Verification items for the finished model (mm, model axes). Give positions to 0.01 mm unless a question says otherwise; leave off trailing zeros. Loops run counter-clockwise (first coordinate to the right, second up) from the corner with the lowest first, then second, coordinate; pieces in that order, holes last. Notation, with made-up numbers: (50, -27) - (64, -27) arc R19 ccw to (64, 7) - close; hole circle Ø7 at (5.25, -32.5). An arc over 180 degrees is marked (long way). Use one line per item in the form item = value.
```python
from build123d import *

# Parameters (mm, degrees)
SKETCH_1_R      = 80.33713036
SKETCH_1_R_2    = 4.1
EXTRUDE_1_DEPTH = 8


with BuildPart() as part:
    # 草图1 → 凸台-拉伸1 (new body)
    with BuildSketch(Plane.XY):
        Circle(SKETCH_1_R)
        with Locations((0, 73.60266962)):
            Circle(SKETCH_1_R_2, mode=Mode.SUBTRACT)
        with Locations((-52.044946802, 52.044946802)):
            Circle(SKETCH_1_R_2, mode=Mode.SUBTRACT)
        with Locations((-73.60266962, 0)):
            Circle(SKETCH_1_R_2, mode=Mode.SUBTRACT)
        with Locations((-52.044946802, -52.044946802)):
            Circle(SKETCH_1_R_2, mode=Mode.SUBTRACT)
        with Locations((0, -73.60266962)):
            Circle(SKETCH_1_R_2, mode=Mode.SUBTRACT)
        with Locations((52.044946802, -52.044946802)):
            Circle(SKETCH_1_R_2, mode=Mode.SUBTRACT)
        with Locations((73.60266962, 0)):
            Circle(SKETCH_1_R_2, mode=Mode.SUBTRACT)
        with Locations((52.044946802, 52.044946802)):
            Circle(SKETCH_1_R_2, mode=Mode.SUBTRACT)
        with Locations((0, 26.022473401)):
            Circle(SKETCH_1_R_2, mode=Mode.SUBTRACT)
        with Locations((22.536123034, -13.0112367)):
            Circle(SKETCH_1_R_2, mode=Mode.SUBTRACT)
        with Locations((-22.536123034, -13.0112367)):
            Circle(SKETCH_1_R_2, mode=Mode.SUBTRACT)
        Circle(SKETCH_1_R_2, mode=Mode.SUBTRACT)
        with BuildLine():
            Line((43.72373161, 48.096104771), (30, 33))
            Line((30, 33), (-30, 33))
            Line((-30, 33), (-43.72373161, 48.096104771))
            ThreePointArc((-43.72373161, 48.096104771), (0, 65), (43.72373161, 48.096104771))
        make_face(mode=Mode.SUBTRACT)
        with BuildLine():
            Line((-64.926428952, -3.091734712), (-44.547727215, -2.121320344))
            Line((-44.547727215, -2.121320344), (-2.121320344, -44.547727215))
            Line((-2.121320344, -44.547727215), (-3.091734712, -64.926428952))
            ThreePointArc((-3.091734712, -64.926428952), (-45.961940777, -45.961940777), (-64.926428952, -3.091734712))
        make_face(mode=Mode.SUBTRACT)
        with BuildLine():
            Line((3.091734712, -64.926428952), (2.121320344, -44.547727215))
            Line((2.121320344, -44.547727215), (44.547727215, -2.121320344))
            Line((44.547727215, -2.121320344), (64.926428952, -3.091734712))
            ThreePointArc((64.926428952, -3.091734712), (45.961940777, -45.961940777), (3.091734712, -64.926428952))
        make_face(mode=Mode.SUBTRACT)
    extrude(amount=EXTRUDE_1_DEPTH)


solid = part.part
```
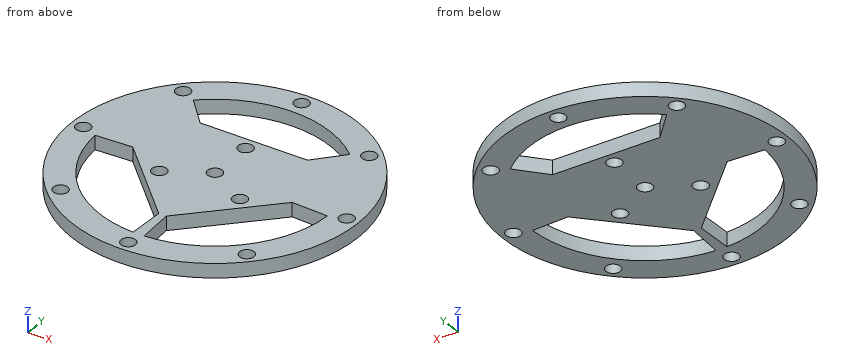
1. Depth check by flat-ended pin: pin 1 Ø2 at (x, z) = (60.5, 4.5) entering from +Y; pin 2 Ø5 at (x, y) = (-52.04, 52.04) entering from -Z; pin 3 Ø3 at (y, z) = (-18.5, 3) entering from +X; pin 4 Ø3 at (x, z) = (-15.5, 2.5) entering from -Y. Enter the tip coordinate at first touch or a pass-through.
Result set:
pin_1 = 53.98
pin_2 = through
pin_3 = 78.52
pin_4 = -79.11
2. Section check C-C, the plane z = 2.25. State how many separate pieces and enclosed holes the cut face has, then the cut area to 3 significant figures.
Result set:
separate_pieces = 1
enclosed_holes = 15
area = 13,300 mm²
3. Section check B-B, the plane y = 0. Record the cut outline in (x, z).
Result set:
outline = (-80.34, 0) - (-77.7, 0) - (-77.7, 8) - (-80.34, 8) - close; (-69.5, 0) - (-4.1, 0) - (-4.1, 8) - (-69.5, 8) - close; (4.1, 0) - (69.5, 0) - (69.5, 8) - (4.1, 8) - close; (77.7, 0) - (80.34, 0) - (80.34, 8) - (77.7, 8) - close
4. Section check A-A, the plane x = 0. Record the cut outline in (y, z), then the cut area to 3 significant figures.
Result set:
outline = (-80.34, 0) - (-77.7, 0) - (-77.7, 8) - (-80.34, 8) - close; (-69.5, 0) - (-4.1, 0) - (-4.1, 8) - (-69.5, 8) - close; (4.1, 0) - (21.92, 0) - (21.92, 8) - (4.1, 8) - close; (30.12, 0) - (33, 0) - (33, 8) - (30.12, 8) - close; (65, 0) - (69.5, 0) - (69.5, 8) - (65, 8) - close; (77.7, 0) - (80.34, 0) - (80.34, 8) - (77.7, 8) - close
area = 767 mm²
5. Scan lines: probe 1 along X at (y, z) = (-38, 1.5); probe 2 along X at (y, z) = (-57.5, 6.75); probe 3 along Y at (x, z) = (23, 3.5). Record each from-to range of solid material in increasing order.
Result set:
probe_1 = -70.78 to -52.74, -8.67 to 8.67, 52.74 to 70.78
probe_2 = -56.11 to -30.31, -2.74 to 2.74, 30.31 to 56.11
probe_3 = -76.97 to -60.79, -23.67 to -17.08, -8.94 to 33, 60.79 to 76.97
6. Section check D-D, the plane y = 59.5. Record the cut outline in (x, z), then the cut area to 3 significant figures.
Result set:
outline = (-53.98, 0) - (-26.17, 0) - (-26.17, 8) - (-53.98, 8) - close; (26.17, 0) - (53.98, 0) - (53.98, 8) - (26.17, 8) - close
area = 445 mm²
